from build123d import *

# Parameters (mm, degrees)
BOSS_EXTRUDE1_DEPTH = 3
SKETCH2_R           = 3
BOSS_EXTRUDE2_DEPTH = 12


with BuildPart() as part:
    # Sketch1 → Boss-Extrude1 (new body)
    with BuildSketch(Plane.XY):
        Polygon((0, -5.773502692), (5, -2.886751346), (5, 2.886751346), (0, 5.773502692), (-5, 2.886751346), (-5, -2.886751346), align=None)
    extrude(amount=BOSS_EXTRUDE1_DEPTH)

    # Sketch2 → Boss-Extrude2 (add)
    with BuildSketch(Plane.XY.offset(3)):
        Circle(SKETCH2_R)
    extrude(amount=BOSS_EXTRUDE2_DEPTH)

    # Sketch3 → Cut-Revolve1 (revolve, cut)
    with BuildSketch(Plane(origin=(0, 0, 0), x_dir=(0, 0, -1), z_dir=(1, 0, 0)), mode=Mode.PRIVATE) as cut_revolve1_sk:
        Polygon((-1, 5.773502692), (0, 5.773502692), (0, 4.773502692), align=None)
    revolve(cut_revolve1_sk.sketch.rotate(Axis((0, 0, 11.168529758), (0, 0, -1)), 90), axis=Axis((0, 0, 11.168529758), (0, 0, -1)), mode=Mode.SUBTRACT)


solid = part.part
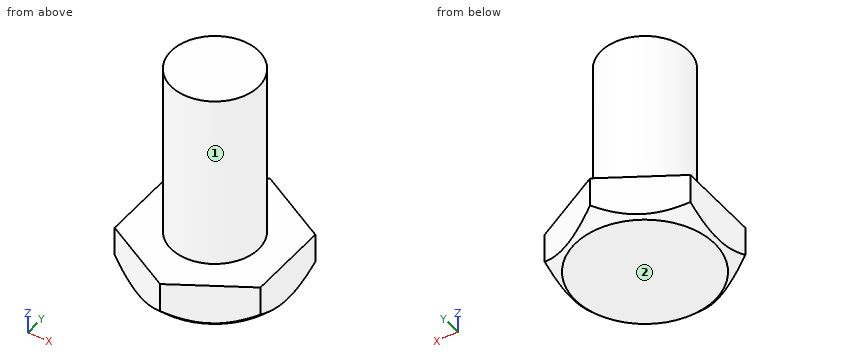
Can you work these out from the model? Positions are in its coordinate system, mm. Face numbers are marked on the shaded views. A direction names the side the tool comes from. Give positions to 0.01 mm unless a question says otherwise; leave off trailing zeros. Loops run counter-clockwise (first coordinate to the right, second up) from the corner with the lowest first, then second, coordinate; pieces in that order, holes last. Notation, with made-up numbers: (55.25, 27.25) - (93.25, 27.25) arc R21 ccw to (93.25, 34.25) - close; hole circle Ø5 at (74.5, -8). An arc over 180 degrees is marked (long way). One line per item, written item: value.
(1) On a 3-axis mill with a long thin cutter (end or side, diameter ignored), from which of +Z, -Z, +X, -X, +Y, -Y can I reach the whole of each face in a straight line? I mean the marked faces 1 and 2. Say none if no direction works.
Verdict:
face 1: +Z
face 2: -Z, +X, -X, +Y, -Y
(2) I'm going to push flat-ended pins straight in: pin 1 (1 mm diameter, centred on x = -3.5, y = 1, fed in from +Z); pin 2 (1 mm diameter, centred on x = 0.5, z = 8.5, fed in from -Y). Where does each tip first touch, or does it pass through?
Verdict:
pin 1: z = 3
pin 2: y = -3
(3) I need wall thicknesses on line 1 along Z through (x, y) = (-3.75, -1.75); line 2 along X through (y, z) = (1.5, 10.75); line 3 along Y through (x, z) = (0.5, 7.25). Which ranges of each line are inside material? Lowest first, please.
Verdict:
line 1: 0 to 3
line 2: -2.6 to 2.6
line 3: -2.96 to 2.96
(4) If we section it at A-A, the plane y = 0: List the corners of the cut face in (x, z) for me.
Verdict:
outline: (-5, 0.23) - (-4.77, 0) - (4.77, 0) - (5, 0.23) - (5, 3) - (3, 3) - (3, 15) - (-3, 15) - (-3, 3) - (-5, 3) - close
(5) If we section it at B-B, the plane z = 14.25: List the corners of the cut face in (x, y) for me.
Verdict:
outline: circle Ø6 at (0, 0)
